```python
from build123d import *

# Parameters (mm, degrees)
SKETCH1_W                  = 95
SKETCH1_H                  = 120
BOSS_EXTRUDE1_DEPTH        = 5
SKETCH2_W                  = 83
SKETCH2_H                  = 5
CUT_EXTRUDE1_DEPTH         = 8
F_4_5_4_5_DIAMETER_HOLE1_D = 4.5


with BuildPart() as part:
    # Sketch1 → Boss-Extrude1 (new body)
    with BuildSketch(Plane(origin=(0, 0, 0), x_dir=(1, 0, 0), z_dir=(0, 1, 0))):
        Rectangle(SKETCH1_W, SKETCH1_H)
    extrude(amount=BOSS_EXTRUDE1_DEPTH)

    # Sketch2 → Cut-Extrude1 (cut)
    with BuildSketch(Plane(origin=(47.5, 0, 0), x_dir=(0, 0, -1), z_dir=(1, 0, 0))):
        with Locations((0, 2.5)):
            Rectangle(SKETCH2_W, SKETCH2_H)
    extrude(amount=-CUT_EXTRUDE1_DEPTH, mode=Mode.SUBTRACT)

    # Ø4.5 (4.5) Diameter Hole1 (through all)
    with Locations(Plane(origin=(0, 5, 0), x_dir=(1, 0, 0), z_dir=(0, 1, 0))):
        with Locations((30.5, 28.5), (27.5, 0), (30.5, -28.5)):
            Hole(F_4_5_4_5_DIAMETER_HOLE1_D / 2)


solid = part.part
```
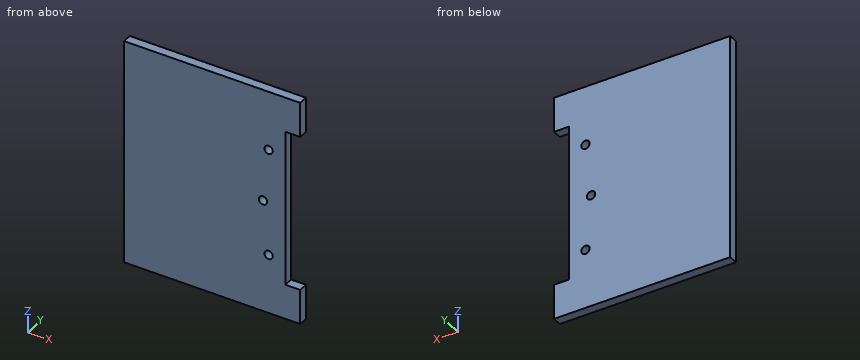
Part model, mm, in its own coordinate system. Coordinates: 2 decimals unless noted, no trailing zeros. Order: outer loops, then holes, each group sorted by start corner. A loop starts at its lowest first (then second) coordinate and runs counter-clockwise, first axis right, second up. Notation, with made-up numbers: (-31, 53) -> (0, 53) arc R22 ccw to (0, 67) -> close; hole circle Ø9 at (-28.75, 78). An arc over 180 degrees is marked (long way). Put each result on its own line as item: value. Start each with the question number.
(1) Pin check, flat tips, straight feed: pin 1 Ø3 at (y, z) = (4, -13.5) entering from +X; pin 2 Ø2.5 at (x, z) = (27.5, 0) entering from +Y. Stop position of each tip, or through.
(2) Band-saw the part on B-B (y = 1.2). Give the cut face in (x, z), then the cut area to 3 significant figures.
(3) Band-saw the part on A-A (z = 28.5). Give the cut face in (x, y), then the cut area to 4 significant figures.
(4) Probe line 1 along Z through (x, y) = (30.5, 2.8); line 2 along X through (y, z) = (2.55, 28.5); line 3 along Z through (x, y) = (27.5, 3.55). List the from-to ranges inside material, lowest first. Write a range as [from, to].
Determined:
1. pin 1: stops at x = 39.5
1. pin 2: passes through
2. outline: (-47.5, -60) -> (47.5, -60) -> (47.5, -41.5) -> (39.5, -41.5) -> (39.5, 41.5) -> (47.5, 41.5) -> (47.5, 60) -> (-47.5, 60) -> close; hole circle Ø4.5 at (27.5, 0); hole circle Ø4.5 at (30.5, -28.5); hole circle Ø4.5 at (30.5, 28.5)
2. area: 10,700 mm²
3. outline: (-47.5, 0) -> (28.25, 0) -> (28.25, 5) -> (-47.5, 5) -> close; (32.75, 0) -> (39.5, 0) -> (39.5, 5) -> (32.75, 5) -> close
3. area: 412.5 mm²
4. line 1: z = [-60, -30.75], [-26.25, 26.25], [30.75, 60]
4. line 2: x = [-47.5, 28.25], [32.75, 39.5]
4. line 3: z = [-60, -2.25], [2.25, 60]
